For this review, take the finished solid that the model builds, in its own axes (mm). A direction names the side the tool comes from. Coordinates: 2 decimals unless noted, no trailing zeros. Loops run counter-clockwise (first coordinate to the right, second up) from the corner with the lowest first, then second, coordinate; pieces in that order, holes last. Notation, with made-up numbers: (67.5, 17) -> (116.5, 17) arc R15 ccw to (116.5, 41) -> close; hole circle Ø10 at (-37, 52.25). An arc over 180 degrees is marked (long way). Answer in a Markdown table with one row per item.
from build123d import *

# Parameters (mm, degrees)
F1_DEPTH = 7
F0_R     = 1.25
F2_DEPTH = 6.4
F3_DEPTH = 2.65
F4_W     = 4.9
F4_H     = 4
F5_DEPTH = 1.9
F6_R     = 2.425
F7_DEPTH = 1.9


with BuildPart() as f1:
    # F0 (on Top) → F1 (new body)
    with BuildSketch(Plane.XY):
        with BuildLine():
            Line((3.52, -11.18), (3.52, 0))
            ThreePointArc((3.52, 0), (1.5919798994, -3.1394266993), (-2.08, -2.8397182959))
            Line((-2.08, -2.8397182959), (-2.08, -7.93))
            Line((-2.08, -7.93), (-4.38, -7.93))
            Line((-4.38, -7.93), (-4.38, -11.18))
            Line((-4.38, -11.18), (0, -11.18))
            Line((0, -11.18), (3.52, -11.18))
        make_face()
    extrude(amount=F1_DEPTH)

    # F0 (on Top) → F2 (join)
    with BuildSketch(Plane.XY):
        with BuildLine():
            ThreePointArc((-2.08, -2.8397182959), (1.5919798994, -3.1394266993), (3.52, 0))
            ThreePointArc((3.52, 0), (-1.5919798994, 3.1394266993), (-2.08, -2.8397182959))
        make_face()
        Circle(F0_R, mode=Mode.SUBTRACT)
    extrude(amount=F2_DEPTH)

    # F0 (on Top) → F3 (join)
    with BuildSketch(Plane.XY):
        Circle(F0_R)
    extrude(amount=F3_DEPTH)

    # F4 (on face) → F5 (cut)
    with BuildSketch(Plane.XZ.offset(11.18)):
        with Locations((-0.43, 3.5)):
            Rectangle(F4_W, F4_H)
    extrude(amount=-F5_DEPTH, mode=Mode.SUBTRACT)

    # F6 (on face) → F7 (cut)
    with BuildSketch(Plane.YZ.offset(3.52)):
        with Locations((-7.255, 3.5)):
            Circle(F6_R)
        with BuildLine():
            ThreePointArc((0, 5.837648391), (-1.78, 3.5), (0, 1.162351609))
            Line((0, 1.162351609), (0, 5.837648391))
        make_face()
        with BuildLine():
            Line((0, 5.837648391), (0, 1.162351609))
            ThreePointArc((0, 1.162351609), (2.1140983629, 1.570654256), (3.07, 3.5))
            ThreePointArc((3.07, 3.5), (2.1140983629, 5.429345744), (0, 5.837648391))
        make_face()
    extrude(amount=-F7_DEPTH, mode=Mode.SUBTRACT)


solid = f1.part
Item 1: For L1, parallel to Y at x = 0, z = 4.45; L2, parallel to Z at x = 1.75, y = -10.25; L3, parallel to Y at x = 2.3, z = 3.5, list the stretches that pass through material, from the lowest coordinate up.
Worked answers:
| item | result |
|---|---|
| L1 | -9.28 to -1.25, 1.25 to 3.52 |
| L2 | 0 to 1.5, 5.5 to 7 |
| L3 | -11.18 to -9.68, -4.83 to -1.78 |
Item 2: For faces 4 (the flat face through (1.62, 1, 4)), 5 (the flat face through (0, -9.28, 4)), 6 (the flat face through (-3, -7.93, 3)), 7 (the cylindrical face through (-0.27, -1.22, 4.5)), list the 3-axis set-ups (+Z, -Z, +X, -X, +Y, -Y) from which the entire face can be reached by the end or side of a thin tool; tool diameter is ignored.
Worked answers:
| item | result |
|---|---|
| face 4 | +X |
| face 5 | -Y |
| face 6 | +Z, -Z, -X |
| face 7 | +Z |
Item 3: Take a section at D-D, the plane x = 2.5. State the section outline as (y, z) points (3 decimals), and give its area (3 significant figures).
Worked answers:
| item | result |
|---|---|
| outline | (-11.18, 0) -> (2.478, 0) -> (2.478, 1.912) arc R2.425 cw (long way) to (2.478, 5.088) -> (2.478, 6.4) -> (-2.478, 6.4) -> (-2.478, 7) -> (-11.18, 7) -> close; hole circle Ø4.85 at (-7.255, 3.5) |
| area | 57.0 mm² |
Item 4: Take a section at B-B, the plane x = 0. State the section outline as (y, z) points, and give its area (3 significant figures).
Worked answers:
| item | result |
|---|---|
| outline | (-11.18, 0) -> (3.52, 0) -> (3.52, 6.4) -> (1.25, 6.4) -> (1.25, 2.65) -> (-1.25, 2.65) -> (-1.25, 6.4) -> (-3.52, 6.4) -> (-3.52, 7) -> (-11.18, 7) -> (-11.18, 5.5) -> (-9.28, 5.5) -> (-9.28, 1.5) -> (-11.18, 1.5) -> close |
| area | 81.7 mm² |
Item 5: Take a section at C-C, the plane y = -5.5. State the section outline as (x, z) points, and give its area (3 significant figures).
Worked answers:
| item | result |
|---|---|
| outline | (-2.08, 0) -> (3.52, 0) -> (3.52, 1.83) -> (1.62, 1.83) -> (1.62, 5.17) -> (3.52, 5.17) -> (3.52, 7) -> (-2.08, 7) -> close |
| area | 32.8 mm² |
Item 6: Take a section at A-A, the plane z = 3.25. State the section outline as (x, y) points, and give its area (3 significant figures).
Worked answers:
| item | result |
|---|---|
| outline | (-4.38, -11.18) -> (-2.88, -11.18) -> (-2.88, -9.28) -> (1.62, -9.28) -> (1.62, -4.84) -> (3.52, -4.84) -> (3.52, -1.77) -> (1.62, -1.77) -> (1.62, 3.06) -> (1.74, 3.06) arc R3.52 ccw to (-2.08, -2.84) -> (-2.08, -7.93) -> (-4.38, -7.93) -> close; (2.02, -11.18) -> (3.52, -11.18) -> (3.52, -9.67) -> (2.02, -9.67) -> close; hole circle Ø2.5 at (0, 0) |
| area | 61.6 mm² |
Item 7: Insertion check: pin 1 (1 mm diameter, centred on y = -4.5, z = 4, fed in from -X); pin 2 (2 mm diameter, centred on x = 0.5, y = 0.5, fed in from +Z); pin 3 (1.2 mm diameter, centred on x = -3.5, z = 2, fed in from +Y). Each pin has a flat end and moves straight along its axis. Give the tip position at first contact, or say it passes through.
Worked answers:
| item | result |
|---|---|
| pin 1 | x = -2.08 |
| pin 2 | z = 6.4 |
| pin 3 | y = 2 |
Item 8: The part is to be moulded in two halves that separate along X. For faces 1 (the flat face through (3.52, -4, 3)), 2 (the cylindrical face through (1.64, -3.115, 6.696)), 3 (the flat face through (-4.38, -10, 3)), say which applies: +X half, -X half, draft (parallel to the pull), parting line (faces both ways), or undercut.
Worked answers:
| item | result |
|---|---|
| face 1 | +X half |
| face 2 | undercut |
| face 3 | -X half |
